from build123d import *

# Parameters (mm, degrees)
F1_DEPTH  = 37
F3_DEPTH  = 37.001
F5_DEPTH  = 37
F7_D      = 3.6
F7_DEPTH  = 10
F7_TIP    = 1.0815491142
F8_D      = 21
F8_DEPTH  = 10
F8_TIP    = 6.3090364998
F9_W      = 11
F9_H      = 5
F10_DEPTH = 37.001
F11_W     = 21
F11_H     = 2
F12_DEPTH = 20
F14_D     = 5.5
F14_DEPTH = 12
F14_TIP   = 1.6523667023


# Not quite as in the source:
# - a feature names something its author has since deleted; it is built from what else it names


with BuildPart() as f1:
    # F0 (on Top) → F1 (new body)
    with BuildSketch(Plane.XY):
        Polygon((-13.5, 27), (-13.5, 0), (-5, 0), (5, 0), (13.5, 0), (13.5, 27), align=None)
    extrude(amount=F1_DEPTH)

    # F2 (on face) → F3 (cut, through all)
    with BuildSketch(Plane.XY.offset(37)):
        Polygon((0, 15.5), (0, 22), (-4, 26), (-10.5, 26), (-10.5, 19.5), (-6.5, 15.5), align=None)
        Polygon((4, 26), (0, 22), (0, 15.5), (6.5, 15.5), (10.5, 19.5), (10.5, 26), align=None)
        Polygon((6.5, 15.5), (0, 15.5), (0, 9), (4, 5), (10.5, 5), (10.5, 11.5), align=None)
        Polygon((0, 9), (0, 15.5), (-6.5, 15.5), (-10.5, 11.5), (-10.5, 5), (-4, 5), align=None)
        Polygon((0, 5), (0, 9), (-4, 5), align=None)
        Polygon((4, 5), (0, 9), (0, 5), align=None)
    extrude(amount=-F3_DEPTH, mode=Mode.SUBTRACT)

    # F4 (on Top) → F5 (join, through all)
    with BuildSketch(Plane.XY):
        Polygon((-13.5, 27), (0, 27), (13.5, 27), (13.5, 0), (19, 0), (19, 51), (-19, 51), (-19, 0), (-13.5, 0), align=None)
        Polygon((15, 30), (0, 30), (-15, 30), (-15, 47), (15, 47), align=None, mode=Mode.SUBTRACT)
    extrude(amount=F5_DEPTH)

    # F7
    with Locations(Plane(origin=(0, 51, 0), x_dir=(-1, 0, 0), z_dir=(0, 1, 0))):
        with Locations((-7.75, 5.0766062413), (7.75, 5.0766062413), (7.75, 31.9233937587), (-7.75, 31.9233937587)):
            Hole(F7_D / 2, depth=F7_DEPTH)
            with Locations((0, 0, -(F7_DEPTH + F7_TIP / 2))):  # 118° drill point
                Cone(0, F7_D / 2, F7_TIP, mode=Mode.SUBTRACT)

    # F8
    with Locations(Plane(origin=(0, 51, 0), x_dir=(-1, 0, 0), z_dir=(0, 1, 0))):
        with Locations((0, 18.5)):
            Hole(F8_D / 2, depth=F8_DEPTH)
            with Locations((0, 0, -(F8_DEPTH + F8_TIP / 2))):  # 118° drill point
                Cone(0, F8_D / 2, F8_TIP, mode=Mode.SUBTRACT)

    # F9 (on face) → F10 (cut, through all)
    with BuildSketch(Plane.XY.offset(37)):
        Polygon((-19, 26), (-19, 0), (-5.5, 0), (-5.5, 5), (-10.5, 5), (-10.5, 11.5), (-6.5, 15.5), (-10.5, 19.5), (-10.5, 26), align=None)
        Polygon((5.5, 5), (5.5, 0), (19, 0), (19, 26), (10.5, 26), (10.5, 19.5), (6.5, 15.5), (10.5, 11.5), (10.5, 5), align=None)
        with Locations((0, 2.5)):
            Rectangle(F9_W, F9_H)
    extrude(amount=-F10_DEPTH, mode=Mode.SUBTRACT)

    # F11 (on face) → F12 (join)
    with BuildSketch(Plane.XY.offset(37)):
        with Locations((0, 27)):
            Rectangle(F11_W, F11_H)
        with Locations((0, 29)):
            Rectangle(F11_W, F11_H)
        Polygon((4, 26), (10.5, 26), (10.5, 28), (-10.5, 28), (-10.5, 26), (-4, 26), align=None)
    extrude(amount=F12_DEPTH)

    # F14
    with Locations(Plane(origin=(0, 30, 0), x_dir=(-1, 0, 0), z_dir=(0, 1, 0))):
        with Locations((0, 47)):
            Hole(F14_D / 2, depth=F14_DEPTH)
            with Locations((0, 0, -(F14_DEPTH + F14_TIP / 2))):  # 118° drill point
                Cone(0, F14_D / 2, F14_TIP, mode=Mode.SUBTRACT)


solid = f1.part
Geometry: final body of the model. Coordinates: model frame, mm. A direction names the side the tool comes from. Give positions to 0.01 mm unless a question says otherwise; leave off trailing zeros. Loops run counter-clockwise (first coordinate to the right, second up) from the corner with the lowest first, then second, coordinate; pieces in that order, holes last. Notation, with made-up numbers: M 84.25,-37 L 94.25,-37 A31 cw 94.25,-9 Z; hole C -19.5,60.25 d3. An arc over 180 degrees is marked long. Put each result on its own line as item: value. Start each with the question number.
1) Cut plane A-A (y = 42.5). Output: boundary loops of the cut face in (x, z), then the cut area to 3 significant figures.
2) Cut plane C-C (x = -7.75). Output: boundary loops of the cut face in (y, z).
3) Contact query for flat-ended pins moving along their axis: pin 1 (4.5 mm diameter, centred on x = 7.75, z = 5.08, fed in from -Y); pin 2 (2 mm diameter, centred on x = -6, z = 46.5, fed in from +Y); pin 3 (2 mm diameter, centred on y = 29, z = 45, fed in from -X); pin 4 (3 mm diameter, centred on x = -6.5, y = 25, fed in from +Z). Output: stop coordinate, or through.
4) Cut plane D-D (z = 35). Output: boundary loops of the cut face in (x, y), then the cut area to 3 significant figures.
5) Pull-direction query (X, two-part tool) for faces 6 (the flat face through (10.5, 28, 47)), 7 (the flat face through (9, 51, 10)), 8 (the flat face through (-15, 38, 18)); classes: pulls with the +X half, pulls with the -X half, needs draft (parallel to the pull), parting line crosses it, or undercut.
6) Ray query, line 1 along X through (y, z) = (42.75, 34); line 2 along Y through (x, z) = (12.5, 25); line 3 along Z through (x, y) = (-7.75, 48). Return the intervals inside material, ascending.
7) Cut plane B-B (z = 45). Output: boundary loops of the cut face in (x, y).
8) Access query for faces 1 (the flat face through (0, 24, 37)), 2 (the flat face through (0, 30, 28)), 3 (the flat face through (-19, 39, 18)), 4 (the flat face through (-10.5, 28, 47)), 5 (the cylindrical face through (-1.37, 48.97, 28.91)). Directions: +Z, -Z, +X, -X, +Y, -Y. A direction counts if a zero-diameter tool reaches every point of the face in a straight line with its end or side. Return the directions, or none.
Verdict:
1. outline: M -19,0 L -15,0 L -15,37 L -19,37 Z; M 15,0 L 19,0 L 19,37 L 15,37 Z
1. area: 296 mm2
2. outline: M 26,0 L 30,0 L 30,57 L 26,57 Z; M 47,0 L 51,0 L 51,3.28 L 47,3.28 Z; M 47,6.88 L 51,6.88 L 51,11.42 L 47,11.42 Z; M 47,25.58 L 51,25.58 L 51,30.12 L 47,30.12 Z; M 47,33.72 L 51,33.72 L 51,37 L 47,37 Z
3. pin 1: y = 26
3. pin 2: y = 30
3. pin 3: x = -10.5
3. pin 4: z = 57
4. outline: M -19,26 L -4,26 L 0,22 L 4,26 L 19,26 L 19,51 L -19,51 Z; hole M -15,30 L 15,30 L 15,47 L -15,47 Z
4. area: 456 mm2
5. face 6: pulls with the +X half
5. face 7: needs draft
5. face 8: undercut
6. line 1: -19 to -15, 15 to 19
6. line 2: 26 to 30, 47 to 51
6. line 3: 0 to 3.28, 6.88 to 11.42, 25.58 to 30.12, 33.72 to 37
7. outline: M -10.5,26 L -1.89,26 L -1.89,30 L -10.5,30 Z; M 1.89,26 L 10.5,26 L 10.5,30 L 1.89,30 Z
8. face 1: +Z, +X, -X, -Y
8. face 2: +Z, -Z
8. face 3: +Z, -Z, -X, +Y, -Y
8. face 4: +Z, -X, +Y, -Y
8. face 5: +Y
